from build123d import *

# Parameters (mm, degrees)
ESTRUSIONE_ESTRUSIONE1_DEPTH = 100
SCHIZZO2_R                   = 0.75
SCHIZZO2_R_2                 = 0.5
TAGLIO_ESTRUSIONE5_DEPTH     = 100
ESTRUSIONE_ESTRUSIONE2_DEPTH = 0.3
ESTRUSIONE_ESTRUSIONE3_START = -0.3
ESTRUSIONE_ESTRUSIONE3_DEPTH = 0.3


with BuildPart() as part:
    # Schizzo1 → Estrusione-Estrusione1 (new body)
    with BuildSketch(Plane.XY):
        with BuildLine():
            Line((-1.5, -18), (-1.2, -18))
            Line((-1.2, -18), (-1.2, -20))
            ThreePointArc((-1.2, -20), (0, -21.2), (1.2, -20))
            Line((1.2, -20), (1.2, -18))
            Line((1.2, -18), (1.5, -18))
            Line((1.5, -18), (1.5, -20))
            ThreePointArc((1.5, -20), (0, -21.5), (-1.5, -20))
            Line((-1.5, -20), (-1.5, -18))
        make_face()
    extrude(amount=ESTRUSIONE_ESTRUSIONE1_DEPTH)

    # Schizzo2 → Taglio-Estrusione5 (cut)
    with BuildSketch(Plane(origin=(1.5, 0, 0), x_dir=(0, 0, -1), z_dir=(1, 0, 0))):
        with Locations(Location((-98.25, -19.75, 0), (0, 0, 340.528779366))):
            Circle(SCHIZZO2_R)
        with Locations(Location((-88.25, -18.95, 0), (0, 0, 90))):
            Circle(SCHIZZO2_R)
        with Locations(Location((-1.75, -19.75, 0), (0, 0, 330))):
            Circle(SCHIZZO2_R_2)
        with BuildLine():
            Line((-98.25, -18), (-98.25, -16.563576213))
            Line((-98.25, -16.563576213), (-100.988318438, -16.563576213))
            Line((-100.988318438, -16.563576213), (-100.988318438, -22.305317171))
            Line((-100.988318438, -22.305317171), (-98.25, -22.305317171))
            Line((-98.25, -22.305317171), (-98.25, -21.5))
            ThreePointArc((-98.25, -21.5), (-100, -19.75), (-98.25, -18))
        make_face()
        with BuildLine():
            Line((-1.75, -18), (-1.75, -17.014244045))
            Line((-1.75, -17.014244045), (0.783864607, -17.014244045))
            Line((0.783864607, -17.014244045), (0.783864607, -22.108114786))
            Line((0.783864607, -22.108114786), (-1.75, -22.108114786))
            Line((-1.75, -22.108114786), (-1.75, -21.5))
            ThreePointArc((-1.75, -21.5), (0, -19.75), (-1.75, -18))
        make_face()
    extrude(amount=-TAGLIO_ESTRUSIONE5_DEPTH, mode=Mode.SUBTRACT)

    # Schizzo3 → Estrusione-Estrusione2 (add)
    with BuildSketch(Plane(origin=(1.5, 0, 0), x_dir=(0, 0, -1), z_dir=(1, 0, 0))):
        with BuildLine():
            Line((-91.25, -18), (-85.25, -18))
            ThreePointArc((-85.25, -18), (-88.25, -17.109772229), (-91.25, -18))
        make_face()
    extrude(amount=-ESTRUSIONE_ESTRUSIONE2_DEPTH)

    # Schizzo4 → Estrusione-Estrusione3 (add)
    with BuildSketch(Plane.ZY.offset(1.5).offset(ESTRUSIONE_ESTRUSIONE3_START)):
        with BuildLine():
            Line((91.25, -18), (85.25, -18))
            ThreePointArc((85.25, -18), (88.25, -17.109772229), (91.25, -18))
        make_face()
    extrude(amount=ESTRUSIONE_ESTRUSIONE3_DEPTH)


solid = part.part
Geometry: final body of the model. Coordinates: model frame, mm. A direction names the side the tool comes from. Round coordinates to 2 decimals unless told otherwise and drop trailing zeros. Loops run counter-clockwise (first coordinate to the right, second up) from the corner with the lowest first, then second, coordinate; pieces in that order, holes last. Notation, with made-up numbers: M -14.75,74 L 20.25,74 A22 ccw 20.25,110 Z; hole C -22,70 d4. An arc over 180 degrees is marked long. Put each result on its own line as item: value. Start each with the question number.
(1) Section query A-A (z = 9). Return loops of the section in (x, y), then the cut area to 3 significant figures.
(2) Material intervals for line 1 along Z through (x, y) = (1.35, -19.75); line 2 along X through (y, z) = (-18.65, 59.5); line 3 along Y through (x, z) = (-1.25, 88.25), sorted ascending. Write a range as [from, to].
(3) Draft query along Y for faces 3 (the face through (1.2, -19, 49)), 4 (the face through (0, -21.5, 49.3)), 5 (the face through (0, -21.2, 49.3)). Return one class per face: +Y half, -Y half, draft (parallel to the pull), parting line (faces both ways), or undercut.
(4) Section query B-B (x = 0). Return loops of the section in (y, z).
(5) Set-up query: faces 1 (the face through (-1.2, -19, 49)), 2 (the face through (-1.5, -19, 49)). Return all of +Z, -Z, +X, -X, +Y, -Y with unobstructed straight access to the full face (end or side cutting, diameter ignored); none if empty.
(6) Contact query for flat-ended pins moving along their axis: pin 1 Ø0.9 at (y, z) = (-19.75, 98.25) entering from -X; pin 2 Ø1 at (x, z) = (-1, 38.5) entering from -Y. Output: stop coordinate, or through.
Findings below:
1. outline: M -1.5,-20 A1.5 ccw 1.5,-20 L 1.5,-18 L 1.2,-18 L 1.2,-20 A1.2 cw -1.2,-20 L -1.2,-18 L -1.5,-18 Z
1. area: 2.47 mm2
2. line 1: z = [0, 1.25], [2.25, 97.5], [99, 100]
2. line 2: x = [-1.5, -1.2], [1.2, 1.5]
2. line 3: y = [-20.83, -19.7], [-18.2, -17.11]
3. face 3: draft
3. face 4: -Y half
3. face 5: +Y half
4. outline: M -21.5,1.75 A1.75 ccw -21.2,0.77 L -21.2,99.23 A1.75 ccw -21.5,98.25 Z
5. face 1: +Z, -Z, +Y
5. face 2: +Z, -Z, -X, +Y, -Y
6. pin 1: passes through
6. pin 2: stops at y = -21.41
